Build history of the part. All positions in model axes, mm. Face numbers are marked on the shaded views. A direction names the side the tool comes from. Round coordinates to 2 decimals unless told otherwise and drop trailing zeros. Write each loop counter-clockwise with the first axis right and the second up, starting at its lowest first coordinate (ties: lowest second). Pieces come first, ordered by that corner, then holes. Notation, with made-up numbers: M -8,85.5 L 29,85.5 A10 ccw 29,92.5 Z; hole C -26.5,34 d11. An arc over 180 degrees is marked long. Write item = value, one per line.
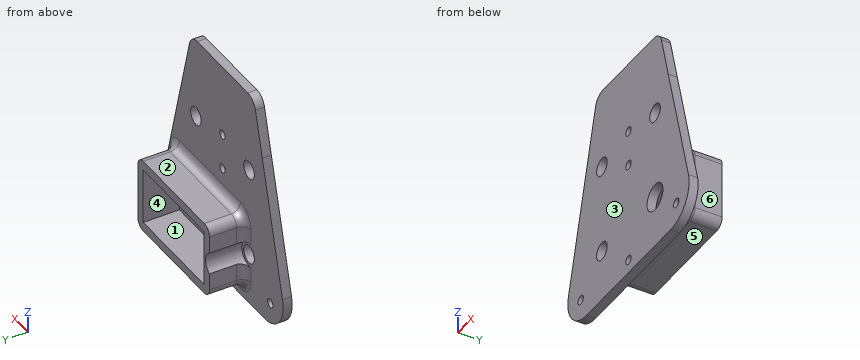
from build123d import *

# Parameters (mm, degrees)
SKETCH1_R               = 3
SKETCH1_R_2             = 2
BOSS_EXTRUDE1_DEPTH     = 2
FILLET1_R               = 7
SKETCH3_W               = 27
SKETCH3_H               = 16.5
SKETCH3_W_2             = 23
SKETCH3_H_2             = 12.5
BOSS_EXTRUDE2_DEPTH     = 8
FILLET2_R               = 2
FILLET3_R               = 2
SKETCH2_R               = 1
CUT_EXTRUDE1_DEPTH      = 2
CUT_EXTRUDE2_DEPTH      = 45.635758586
CUT_EXTRUDE2_DEPTH_BACK = 45.635758586
SKETCH4_R               = 2
SKETCH5_R               = 2.75
CUT_EXTRUDE3_DEPTH      = 45.635758586
FILLET4_R               = 3


with BuildPart() as part:
    # Sketch1 → Boss-Extrude1 (new body)
    with BuildSketch(Plane(origin=(0, 0, 0), x_dir=(1, 0, 0), z_dir=(0, 1, 0))):
        Polygon((15, 0), (24.948794511, 37.5), (-24.948794511, 37.5), (-15, 0), (-11.816385757, -12), (11.816385757, -12), align=None)
        with Locations(Location((10, 26, 0), (0, 0, 270))):
            Circle(SKETCH1_R, mode=Mode.SUBTRACT)
        with Locations(Location((10, 6, 0), (0, 0, 270))):
            Circle(SKETCH1_R_2, mode=Mode.SUBTRACT)
        with Locations(Location((-10, 6, 0), (0, 0, 90))):
            Circle(SKETCH1_R_2, mode=Mode.SUBTRACT)
    extrude(amount=BOSS_EXTRUDE1_DEPTH)

    # Fillet1
    fillet1_edges = [part.edges().sort_by_distance(p)[0] for p in [
        (-24.948794511, 1, -37.5),
        (24.948794511, 1, -37.5),
    ]]
    fillet(fillet1_edges, radius=FILLET1_R)

    # Sketch3 → Boss-Extrude2 (add)
    with BuildSketch(Plane(origin=(0, 2, 0), x_dir=(1, 0, 0), z_dir=(0, 1, 0))):
        with Locations((4.75, 26)):
            Rectangle(SKETCH3_W, SKETCH3_H)
        with Locations((4.75, 26)):
            Rectangle(SKETCH3_W_2, SKETCH3_H_2, mode=Mode.SUBTRACT)
    extrude(amount=BOSS_EXTRUDE2_DEPTH)

    # Fillet2
    fillet2_edges = [part.edges().sort_by_distance(p)[0] for p in [
        (-8.75, 6, -34.25),
        (-8.75, 6, -17.75),
        (18.25, 6, -17.75),
        (18.25, 6, -34.25),
    ]]
    fillet(fillet2_edges, radius=FILLET2_R)

    # Fillet3
    fillet3_edges = [part.edges().sort_by_distance(p)[0] for p in [
        (4.75, 2, -17.75),
        (-8.75, 2, -26),
        (18.25, 2, -26),
        (4.75, 2, -34.25),
        (-8.164213562, 2, -18.335786438),
        (17.664213562, 2, -18.335786438),
        (17.664213562, 2, -33.664213562),
        (-8.164213562, 2, -33.664213562),
    ]]
    fillet(fillet3_edges, radius=FILLET3_R)

    # Sketch2 → Cut-Extrude1 (cut)
    with BuildSketch(Plane(origin=(0, 2, 0), x_dir=(1, 0, 0), z_dir=(0, 1, 0))):
        with Locations(Location((0, 34.5, 0), (0, 0, 270))):
            Circle(SKETCH2_R)
        with Locations(Location((18, 32.5, 0), (0, 0, 270))):
            Circle(SKETCH2_R)
        with Locations(Location((0, 4, 0), (0, 0, 270))):
            Circle(SKETCH2_R)
        with Locations(Location((0, 12, 0), (0, 0, 270))):
            Circle(SKETCH2_R)
        with Locations(Location((-18, 32.5, 0), (0, 0, 90))):
            Circle(SKETCH2_R)
    extrude(amount=-CUT_EXTRUDE1_DEPTH, mode=Mode.SUBTRACT)

    # Sketch4 → Cut-Extrude2 (cut, two sides: drawn at the far end of the back side and taken through both)
    with BuildSketch(Plane(origin=(0, 2, 0), x_dir=(1, 0, 0), z_dir=(0, 1, 0)).offset(-CUT_EXTRUDE2_DEPTH_BACK)):
        with Locations(Location((-10, 26, 0), (0, 0, 270))):
            Circle(SKETCH4_R)
    extrude(amount=CUT_EXTRUDE2_DEPTH + CUT_EXTRUDE2_DEPTH_BACK, mode=Mode.SUBTRACT)

    # Sketch5 → Cut-Extrude3 (cut, through all)
    with BuildSketch(Plane(origin=(0, 2, 0), x_dir=(1, 0, 0), z_dir=(0, 1, 0))):
        with Locations((-10, 26)):
            Circle(SKETCH5_R)
    extrude(amount=CUT_EXTRUDE3_DEPTH, mode=Mode.SUBTRACT)

    # Fillet4
    fillet4_edges = [part.edges().sort_by_distance(p)[0] for p in [
        (11.816385757, 1, 12),
        (-11.816385757, 1, 12),
    ]]
    fillet(fillet4_edges, radius=FILLET4_R)


solid = part.part
1. Probe probe 1 along X at (y, z) = (1.4, -26); probe 2 along Z at (x, y) = (-10, 1.1); probe 3 along Z at (x, y) = (6, 8.75). List the from-to ranges inside material, lowest first.
Responses:
probe_1 = -21.9 to -12, -8 to 7, 13 to 21.9
probe_2 = -37.5 to -28, -24 to -8, -4 to 11.96
probe_3 = -34.25 to -32.25, -19.75 to -17.75
2. Band-saw the part on D-D (z = -6). List the corners of the cut face in (x, y), plus the area to 3 significant figures.
Responses:
outline = M -16.59,0 L -12,0 L -12,2 L -16.59,2 Z; M -8,0 L 8,0 L 8,2 L -8,2 Z; M 12,0 L 16.59,0 L 16.59,2 L 12,2 Z
area = 50.4 mm²
3. Tool access for the marked faces 1, 2 and 3: list every direction of +Z, -Z, +X, -X, +Y, -Y with a clear straight run to the whole face (end or side of a thin tool).
Responses:
face_1 = +Y
face_2 = +Z, +X, -X, +Y
face_3 = +Z, -Z, +X, -X, -Y
4. Flat gauge pins, fed straight in: pin 1 (2.5 mm diameter, centred on x = 9, y = 6, fed in from -Z); pin 2 (1.2 mm diameter, centred on x = -18, z = -32.5, fed in from -Y); pin 3 (1.5 mm diameter, centred on y = 4.5, z = -28.5, fed in from +X); pin 4 (5 mm diameter, centred on x = -10, z = -26, fed in from +Y). Where does each tip first touch, or does it go through?
Responses:
pin_1 = -34.25
pin_2 = through
pin_3 = 18.27
pin_4 = 2
5. Mould opens along X. For the marked faces 4, 5 and 6 say: pulls with the +X half, pulls with the -X half, needs draft (parallel to the pull), parting line crosses it, or undercut.
Responses:
face_4 = undercut
face_5 = needs draft
face_6 = pulls with the +X half
6. Band-saw the part on B-B (y = 9.25). List the corners of the cut face in (x, z), plus the area to 3 significant figures.
Responses:
outline = M -8.75,-32.25 A2 ccw -6.75,-34.25 L 16.25,-34.25 A2 ccw 18.25,-32.25 L 18.25,-19.75 A2 ccw 16.25,-17.75 L -6.75,-17.75 A2 ccw -8.75,-19.75 L -8.75,-23.55 A2.75 cw -8.75,-28.45 Z; hole M -6.75,-32.25 L 16.25,-32.25 L 16.25,-19.75 L -6.75,-19.75 Z
area = 149 mm²
7. Band-saw the part on A-A (z = -12). List the corners of the cut face in (x, y), plus the area to 3 significant figures.
Responses:
outline = M -18.18,0 L -1,0 L -1,2 L -18.18,2 Z; M 1,0 L 18.18,0 L 18.18,2 L 1,2 Z
area = 68.7 mm²
8. Band-saw the part on C-C (x = -18). List the corners of the cut face in (y, z).
Responses:
outline = M 0,-37.16 L 2,-37.16 L 2,-33.5 L 0,-33.5 Z; M 0,-31.5 L 2,-31.5 L 2,-11.31 L 0,-11.31 Z
